Design review of the part built by this model. Coordinates are the model's own, in mm. A direction names the side the tool comes from. Coordinates: 2 decimals unless noted, no trailing zeros. Loops run counter-clockwise (first coordinate to the right, second up) from the corner with the lowest first, then second, coordinate; pieces in that order, holes last. Notation, with made-up numbers: (49, -26) -> (93, -26) arc R17 cw to (93, -22) -> close; hole circle Ø6 at (73, 74). An arc over 180 degrees is marked (long way). Use one line per item in the form item = value. Start each with the question number.
1. Wall thickness on line 1 (Z direction, x = 0.2, y = 11.25); line 2 (Y direction, x = 0.9, z = 0.2); line 3 (Z direction, x = 1.1, y = 11): over which ranges is each line inside the solid? List them lowest first. Write a range as from..to.
2. Machinability: for faces 1 (the face through (-1, 10.1, 1)), 2 (the face through (0, 0, 0)), which of the approach directions +Z, -Z, +X, -X, +Y, -Y give a long, thin tool a straight path to every point of the face, cutting with its end or side? Answer none if there is none.
3. For pin 1 (1.5 mm diameter, centred on x = -1, y = 2.5, fed in from +Z); pin 2 (1 mm diameter, centred on y = 2, z = -1, fed in from +X), all flat-tipped, find the tip position at first contact; note any pin that passes through.
4. Consider section A-A (y = 2). State the section outline as (x, z) points.
from build123d import *

# Parameters (mm, degrees)
FILLET_1_R          = 0.1
SKETCH_2_W          = 3
SKETCH_2_H          = 0.7
CUT_EXTRUDE_1_DEPTH = 0.7


with BuildPart() as part:
    # Sketch 1 → Revolve 1 (revolve)
    with BuildSketch(Plane.XY, mode=Mode.PRIVATE) as revolve_1_sk:
        with BuildLine():
            Line((1.9, 10.1), (1, 10.1))
            Line((1, 10.1), (1, 0.3))
            Line((1, 0.3), (0.7, 0))
            Line((0.7, 0), (0, 0))
            Line((0, 0), (0, 11.5))
            Line((0, 11.5), (0.7, 11.5))
            ThreePointArc((0.7, 11.5), (1.445839439, 10.925005233), (1.9, 10.1))
        make_face()
    revolve(revolve_1_sk.sketch.rotate(Axis((0, 0, 0), (0, 1, 0)), 90), axis=Axis((0, 0, 0), (0, 1, 0)))

    # Fillet 1
    fillet_1_edges = [part.edges().sort_by_distance(p)[0] for p in [
        (0, 10.1, 1.9),
    ]]
    fillet(fillet_1_edges, radius=FILLET_1_R)

    # Sketch 2 → Cut-Extrude 1 (cut)
    with BuildSketch(Plane(origin=(0, 11.5, 0), x_dir=(-1, 0, 0), z_dir=(0, 1, 0))):
        Rectangle(SKETCH_2_W, SKETCH_2_H)
    extrude(amount=-CUT_EXTRUDE_1_DEPTH, mode=Mode.SUBTRACT)


solid = part.part
Geometry check:
q1.line_1 = -1.09..-0.35, 0.35..1.09
q1.line_2 = 0.22..10.8
q1.line_3 = -0.83..-0.35, 0.35..0.83
q2.face_1 = -Y
q2.face_2 = +Z, -Z, +X, -X, -Y
q3.pin_1 = 0.97
q3.pin_2 = 0.87
q4.outline = circle Ø2 at (0, 0)
